Check sheet for the modelled part. Datum: model origin and axes. Units: mm. Face numbers are marked on the shaded views. Round coordinates to 2 decimals unless told otherwise and drop trailing zeros. Order: outer loops, then holes, each group sorted by start corner. A loop starts at its lowest first (then second) coordinate and runs counter-clockwise, first axis right, second up. Notation, with made-up numbers: (-2, 60) -> (54, 60) arc R34 ccw to (54, 91) -> close; hole circle Ø4 at (40.25, 63.5). An arc over 180 degrees is marked (long way). Answer in a Markdown table with one row per item.
from build123d import *

# Parameters (mm, degrees)
F1_DEPTH = 50.8


with BuildPart() as f1:
    # F0 (on Front) → F1 (new body, symmetric)
    with BuildSketch(Plane.XZ):
        with BuildLine():
            ThreePointArc((-79.9545346996, -72.4959198801), (-67.2545346996, -72.4959198801), (-60.9045346996, -83.4944425082))
            Line((-60.9045346996, -83.4944425082), (-41.8545346996, -83.4944425082))
            ThreePointArc((-41.8545346996, -83.4944425082), (-57.7295346996, -55.998135938), (-89.4795346996, -55.998135938))
            Line((-89.4795346996, -55.998135938), (-79.9545346996, -72.4959198801))
        make_face()
        with BuildLine():
            Line((-41.8545346996, -83.4944425082), (-60.9045346996, -83.4944425082))
            ThreePointArc((-60.9045346996, -83.4944425082), (-79.9545346996, -94.4929651363), (-79.9545346996, -72.4959198801))
            Line((-79.9545346996, -72.4959198801), (-89.4795346996, -55.998135938))
            ThreePointArc((-89.4795346996, -55.998135938), (-89.4795346996, -110.9907490783), (-41.8545346996, -83.4944425082))
        make_face()
        with BuildLine():
            ThreePointArc((-89.4795346996, -55.998135938), (-57.7295346996, -55.998135938), (-41.8545346996, -83.4944425082))
            Line((-41.8545346996, -83.4944425082), (47.0454653004, -83.4944425082))
            ThreePointArc((47.0454653004, -83.4944425082), (62.9204653004, -55.998135938), (94.6704653004, -55.998135938))
            Line((94.6704653004, -55.998135938), (161.9071689529, 60.4592509217))
            ThreePointArc((161.9071689529, 60.4592509217), (150.2858623828, 72.0805574918), (146.0321689529, 87.9555574918))
            Line((146.0321689529, 87.9555574918), (-140.8412383522, 87.9555574918))
            ThreePointArc((-140.8412383522, 87.9555574918), (-145.094931782, 72.0805574918), (-156.7162383522, 60.4592509217))
            Line((-156.7162383522, 60.4592509217), (-89.4795346996, -55.998135938))
        make_face()
        with BuildLine():
            ThreePointArc((94.6704653004, -55.998135938), (62.9204653004, -55.998135938), (47.0454653004, -83.4944425082))
            Line((47.0454653004, -83.4944425082), (66.0954653004, -83.4944425082))
            ThreePointArc((66.0954653004, -83.4944425082), (72.4454653004, -72.4959198801), (85.1454653004, -72.4959198801))
            Line((85.1454653004, -72.4959198801), (94.6704653004, -55.998135938))
        make_face()
        with BuildLine():
            Line((66.0954653004, -83.4944425082), (47.0454653004, -83.4944425082))
            ThreePointArc((47.0454653004, -83.4944425082), (78.7954653004, -115.2444425082), (110.5454653004, -83.4944425082))
            ThreePointArc((110.5454653004, -83.4944425082), (106.2917718705, -67.6194425082), (94.6704653004, -55.998135938))
            Line((94.6704653004, -55.998135938), (85.1454653004, -72.4959198801))
            ThreePointArc((85.1454653004, -72.4959198801), (89.7939879284, -77.1444425082), (91.4954653004, -83.4944425082))
            ThreePointArc((91.4954653004, -83.4944425082), (78.7954653004, -96.1944425082), (66.0954653004, -83.4944425082))
        make_face()
        with BuildLine():
            ThreePointArc((-140.8412383522, 87.9555574918), (-200.0875449223, 103.8305574918), (-156.7162383522, 60.4592509217))
            Line((-156.7162383522, 60.4592509217), (-166.2412383522, 76.9570348637))
            ThreePointArc((-166.2412383522, 76.9570348637), (-183.5897609803, 94.3055574918), (-159.8912383522, 87.9555574918))
            Line((-159.8912383522, 87.9555574918), (-140.8412383522, 87.9555574918))
        make_face()
        with BuildLine():
            Line((-166.2412383522, 76.9570348637), (-156.7162383522, 60.4592509217))
            ThreePointArc((-156.7162383522, 60.4592509217), (-145.094931782, 72.0805574918), (-140.8412383522, 87.9555574918))
            Line((-140.8412383522, 87.9555574918), (-159.8912383522, 87.9555574918))
            ThreePointArc((-159.8912383522, 87.9555574918), (-161.5927157241, 81.6055574918), (-166.2412383522, 76.9570348637))
        make_face()
        with BuildLine():
            ThreePointArc((146.0321689529, 87.9555574918), (150.2858623828, 72.0805574918), (161.9071689529, 60.4592509217))
            Line((161.9071689529, 60.4592509217), (171.4321689529, 76.9570348637))
            ThreePointArc((171.4321689529, 76.9570348637), (166.7836463249, 81.6055574918), (165.0821689529, 87.9555574918))
            Line((165.0821689529, 87.9555574918), (146.0321689529, 87.9555574918))
        make_face()
        with BuildLine():
            Line((171.4321689529, 76.9570348637), (161.9071689529, 60.4592509217))
            ThreePointArc((161.9071689529, 60.4592509217), (193.6571689529, 60.4592509217), (209.5321689529, 87.9555574918))
            ThreePointArc((209.5321689529, 87.9555574918), (177.7821689529, 119.7055574918), (146.0321689529, 87.9555574918))
            Line((146.0321689529, 87.9555574918), (165.0821689529, 87.9555574918))
            ThreePointArc((165.0821689529, 87.9555574918), (177.7821689529, 100.6555574918), (190.4821689529, 87.9555574918))
            ThreePointArc((190.4821689529, 87.9555574918), (184.1321689529, 76.9570348637), (171.4321689529, 76.9570348637))
        make_face()
    extrude(amount=F1_DEPTH, both=True)


solid = f1.part
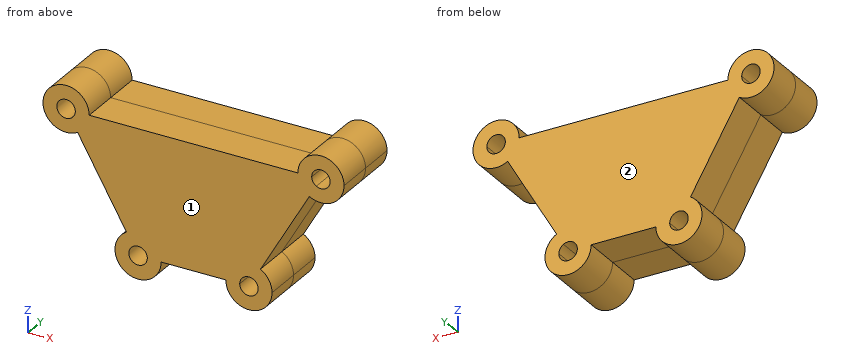
Item 1: Cross-section at A-A (z = -89.5). Record the boundary of the cut face in (x, y), and give its area (3 significant figures).
Result sheet:
| item | result |
|---|---|
| outline | (-104.78, -50.8) -> (-84.79, -50.8) -> (-84.79, 50.8) -> (-104.78, 50.8) -> close; (-62.41, -50.8) -> (-42.43, -50.8) -> (-42.43, 50.8) -> (-62.41, 50.8) -> close; (47.62, -50.8) -> (67.61, -50.8) -> (67.61, 50.8) -> (47.62, 50.8) -> close; (89.99, -50.8) -> (109.97, -50.8) -> (109.97, 50.8) -> (89.99, 50.8) -> close |
| area | 8,120 mm^2 |
Item 2: Cross-section at D-D (x = -16). Record the boundary of the cut face in (y, z), and give its area (3 significant figures).
Result sheet:
| item | result |
|---|---|
| outline | (-50.8, -83.49) -> (50.8, -83.49) -> (50.8, 87.96) -> (-50.8, 87.96) -> close |
| area | 17,400 mm^2 |
Item 3: Cross-section at C-C (x = -74). Record the boundary of the cut face in (y, z), and give its area (3 significant figures).
Result sheet:
| item | result |
|---|---|
| outline | (-50.8, -115.24) -> (50.8, -115.24) -> (50.8, -96.19) -> (-50.8, -96.19) -> close; (-50.8, -70.8) -> (50.8, -70.8) -> (50.8, 87.96) -> (-50.8, 87.96) -> close |
| area | 18,100 mm^2 |
Item 4: Cross-section at B-B (y = -36.5). Record the boundary of the cut face in (x, z).
Result sheet:
| item | result |
|---|---|
| outline | (-156.72, 60.46) -> (-89.48, -56) arc R31.75 ccw (long way) to (-41.85, -83.49) -> (47.05, -83.49) arc R31.75 ccw (long way) to (94.67, -56) -> (161.91, 60.46) arc R31.75 ccw (long way) to (146.03, 87.96) -> (-140.84, 87.96) arc R31.75 ccw (long way) to start; hole circle Ø25.4 at (-172.59, 87.96); hole circle Ø25.4 at (-73.6, -83.49); hole circle Ø25.4 at (78.8, -83.49); hole circle Ø25.4 at (177.78, 87.96) |
Item 5: Mould release check, pull along Y, two halves, no side actions. Record for the marked faces 1 and 2: pulls with the +Y half, pulls with the -Y half, needs draft (parallel to the pull), parting line crosses it, or undercut.
Result sheet:
| item | result |
|---|---|
| face 1 | pulls with the -Y half |
| face 2 | pulls with the +Y half |
Item 6: Depth check by flat-ended pin: P1, Ø1, axis at y = 39, z = -2.5, coming from the +X side; P2, Ø1.5, axis at y = -13.5, z = 62.5, coming from the +X side; P3, Ø5, axis at x = -111, y = 29, coming from the -Z side. Enter the tip coordinate at first touch or a pass-through.
Result sheet:
| item | result |
|---|---|
| P1 | stops at x = 125.85 |
| P2 | stops at x = 197.72 |
| P3 | stops at z = -23.05 |
Item 7: Scan lines: line 1 (X direction, y = -17, z = -85); line 2 (X direction, y = -38, z = 85.5); line 3 (X direction, y = 30, z = 82.5). Record each from-to range of solid material in increasing order. Write a range as [from, to].
Result sheet:
| item | result |
|---|---|
| line 1 | x = [-105.32, -86.21], [-60.99, -41.89], [47.08, 66.19], [91.41, 110.51] |
| line 2 | x = [-204.25, -185.05], [-160.13, 165.32], [190.24, 209.44] |
| line 3 | x = [-203.87, -184.06], [-161.12, 166.31], [189.25, 209.06] |
